Could you check a few things on this model? Use its own coordinates, in mm. Face numbers are marked on the shaded views. A direction names the side the tool comes from. Give positions to 0.01 mm unless a question says otherwise; leave off trailing zeros. Order: outer loops, then holes, each group sorted by start corner. A loop starts at its lowest first (then second) coordinate and runs counter-clockwise, first axis right, second up. Notation, with made-up numbers: (-21.75, 12) - (11.25, 12) arc R19 ccw to (11.25, 23) - close; hole circle Ø9 at (52.5, -8.75). An arc over 180 degrees is marked (long way). Put each result on its own line as item: value.
from build123d import *

# Parameters (mm, degrees)
CYLINDER060_R     = 4
CYLINDER060_DEPTH = 10
BOX018_W          = 6.3
BOX018_H          = 1.8
BOX018_DEPTH      = 14.2
ARRAY003_COUNT    = 16
CYLINDER056_R     = 10.8
CYLINDER056_DEPTH = 14.2
BOX015_W          = 14
BOX015_H          = 54
BOX015_DEPTH      = 15
BOX016_W          = 40
BOX016_H          = 40
BOX016_DEPTH      = 10
PRISM008_DEPTH    = 2.4
PRISM001_DEPTH    = 2.4
CYLINDER012_R     = 1.25
CYLINDER012_DEPTH = 50
CYLINDER011_R     = 1.25
CYLINDER011_DEPTH = 50
CYLINDER007_R     = 6.75
CYLINDER007_DEPTH = 50
CYLINDER008_R     = 6.75
CYLINDER008_DEPTH = 50
BOX013_W          = 18
BOX013_H          = 18
BOX013_DEPTH      = 15
BOX003_W          = 18
BOX003_H          = 18
BOX003_DEPTH      = 15
CYLINDER004_R     = 11.2
CYLINDER004_DEPTH = 23
CYLINDER002_R     = 0.9
CYLINDER002_DEPTH = 19.75
ARRAY002_COUNT    = 10
CYLINDER006_R     = 10.5
CYLINDER006_DEPTH = 32
CYLINDER005_R     = 20
CYLINDER005_DEPTH = 15
FILLET003_R       = 1
CYLINDER051_R     = 1.25
CYLINDER051_DEPTH = 50
BOX011_W          = 16
BOX011_H          = 1
BOX011_DEPTH      = 15
CYLINDER052_R     = 1.25
CYLINDER052_DEPTH = 50
BOX012_W          = 16
BOX012_H          = 1
BOX012_DEPTH      = 15
FILLET010_R       = 0.9
CYLINDER053_R     = 10.5
CYLINDER053_DEPTH = 15
PAD_DEPTH         = 50
BOX014_W          = 10
BOX014_H          = 54
BOX014_DEPTH      = 15
FILLET011_R       = 2


with BuildPart() as cylinder055:
    # Cylinder060 → Cylinder060 (new body)
    with BuildSketch(Plane.XY.offset(21.7)):
        Circle(CYLINDER060_R)
    extrude(amount=CYLINDER060_DEPTH)


with BuildPart() as array003:
    # Box018 → Box018 (new body)
    with BuildSketch(Plane(origin=(6, -0.9, 15), x_dir=(1, 0, 0), z_dir=(0, 0, 1))):
        with Locations((3.15, 0.9)):
            Rectangle(BOX018_W, BOX018_H)
    extrude(amount=BOX018_DEPTH)

    # Array003: Array003 ×16 about axis
    array003_axis = Axis((0, 0, 0), (0, 0, 1))


with BuildPart() as array003_1:
    add(array003.part)
    for i in range(1, ARRAY003_COUNT):
        add(array003.part.rotate(array003_axis, i * 360 / ARRAY003_COUNT))


with BuildPart() as fusion020:
    # Cylinder056 → Cylinder056 (new body)
    with BuildSketch(Plane.XY.offset(15)):
        Circle(CYLINDER056_R)
    extrude(amount=CYLINDER056_DEPTH)

    # Fusion020: union Array003
    add(array003_1.part)


with BuildPart() as cube015:
    # Box015 → Box015 (new body)
    with BuildSketch(Plane(origin=(15, -27, 15), x_dir=(1, 0, 0), z_dir=(0, 0, 1))):
        with Locations((7, 27)):
            Rectangle(BOX015_W, BOX015_H)
    extrude(amount=BOX015_DEPTH)


with BuildPart() as cube016:
    # Box016 → Box016 (new body)
    with BuildSketch(Plane(origin=(-20, -20, 5), x_dir=(1, 0, 0), z_dir=(0, 0, 1))):
        with Locations((20, 20)):
            Rectangle(BOX016_W, BOX016_H)
    extrude(amount=BOX016_DEPTH)


with BuildPart() as prism008:
    # Prism008 → Prism008 (new body)
    with BuildSketch(Plane(origin=(0, 28, 22.5), x_dir=(1, 0, 0), z_dir=(0, -1, 0))):
        Polygon((3.15, 0), (1.575, 2.72798), (-1.575, 2.72798), (-3.15, 0), (-1.575, -2.72798), (1.575, -2.72798), align=None)
    extrude(amount=PRISM008_DEPTH)


with BuildPart() as prism001:
    # Prism001 → Prism001 (new body)
    with BuildSketch(Plane(origin=(0, -25.5, 22.5), x_dir=(1, 0, 0), z_dir=(0, -1, 0))):
        Polygon((3.15, 0), (1.575, 2.72798), (-1.575, 2.72798), (-3.15, 0), (-1.575, -2.72798), (1.575, -2.72798), align=None)
    extrude(amount=PRISM001_DEPTH)


with BuildPart() as cylinder011:
    # Cylinder012 → Cylinder012 (new body)
    with BuildSketch(Plane(origin=(0, 69, 22.5), x_dir=(1, 0, 0), z_dir=(0, -1, 0))):
        Circle(CYLINDER012_R)
    extrude(amount=CYLINDER012_DEPTH)


with BuildPart() as cylinder010:
    # Cylinder011 → Cylinder011 (new body)
    with BuildSketch(Plane(origin=(0, -16, 22.5), x_dir=(1, 0, 0), z_dir=(0, -1, 0))):
        Circle(CYLINDER011_R)
    extrude(amount=CYLINDER011_DEPTH)


with BuildPart() as cylinder007:
    # Cylinder007 → Cylinder007 (new body)
    with BuildSketch(Plane(origin=(-24, 19, 22.5), x_dir=(0, 0, -1), z_dir=(1, 0, 0))):
        Circle(CYLINDER007_R)
    extrude(amount=CYLINDER007_DEPTH)


with BuildPart() as cylinder008:
    # Cylinder008 → Cylinder008 (new body)
    with BuildSketch(Plane(origin=(-24, -19, 22.5), x_dir=(0, 0, -1), z_dir=(1, 0, 0))):
        Circle(CYLINDER008_R)
    extrude(amount=CYLINDER008_DEPTH)


with BuildPart() as cube013:
    # Box013 → Box013 (new body)
    with BuildSketch(Plane(origin=(-9, -29, 15), x_dir=(1, 0, 0), z_dir=(0, 0, 1))):
        with Locations((9, 9)):
            Rectangle(BOX013_W, BOX013_H)
    extrude(amount=BOX013_DEPTH)


with BuildPart() as cube003:
    # Box003 → Box003 (new body)
    with BuildSketch(Plane(origin=(-9, 11, 15), x_dir=(1, 0, 0), z_dir=(0, 0, 1))):
        with Locations((9, 9)):
            Rectangle(BOX003_W, BOX003_H)
    extrude(amount=BOX003_DEPTH)


with BuildPart() as cylinder004:
    # Cylinder004 → Cylinder004 (new body)
    with BuildSketch(Plane.XY):
        Circle(CYLINDER004_R)
    extrude(amount=CYLINDER004_DEPTH)


with BuildPart() as obj1:
    # Cylinder002 → Cylinder002 (new body)
    with BuildSketch(Plane(origin=(0, 0, 15), x_dir=(0, 0, -1), z_dir=(1, 0, 0))):
        Circle(CYLINDER002_R)
    extrude(amount=CYLINDER002_DEPTH)

    # Array002: obj1 ×10 about axis
    array002_axis = Axis((0, 0, 0), (0, 0, 1))


with BuildPart() as obj1_1:
    add(obj1.part)
    for i in range(1, ARRAY002_COUNT):
        add(obj1.part.rotate(array002_axis, i * 360 / ARRAY002_COUNT))

    # Cut002: cut Cylinder004
    add(cylinder004.part, mode=Mode.SUBTRACT)


with BuildPart() as cylinder006:
    # Cylinder006 → Cylinder006 (new body)
    with BuildSketch(Plane.XY):
        Circle(CYLINDER006_R)
    extrude(amount=CYLINDER006_DEPTH)


with BuildPart() as obj2:
    # Cylinder005 → Cylinder005 (new body)
    with BuildSketch(Plane.XY.offset(15)):
        Circle(CYLINDER005_R)
    extrude(amount=CYLINDER005_DEPTH)

    # Cut004: cut Cylinder006
    add(cylinder006.part, mode=Mode.SUBTRACT)

    # Fusion001: union obj1
    add(obj1_1.part)

    # Fusion002: union Cube013, Cube003
    add(cube013.part)
    add(cube003.part)

    # Cut005: cut Cylinder008
    add(cylinder008.part, mode=Mode.SUBTRACT)

    # Cut006: cut Cylinder007
    add(cylinder007.part, mode=Mode.SUBTRACT)

    # Fillet003
    fillet003_edges = [obj2.edges().sort_by_distance(p)[0] for p in [
        (-9, -17.860571, 29.576567),
        (-9, -17.860571, 15.423433),
        (-9, -29, 22.5),
        (-9, 17.860571, 15.423433),
        (-9, 17.860571, 29.576567),
        (9, -29, 22.5),
        (9, -17.860571, 29.576567),
        (9, -17.860571, 15.423433),
        (9, 17.860571, 29.576567),
        (9, 17.860571, 15.423433),
        (9, 29, 22.5),
        (-9, 29, 22.5),
    ]]
    fillet(fillet003_edges, radius=FILLET003_R)

    # Cut008: cut Cylinder010
    add(cylinder010.part, mode=Mode.SUBTRACT)

    # Cut009: cut Cylinder011
    add(cylinder011.part, mode=Mode.SUBTRACT)

    # Cut035: cut Prism001
    add(prism001.part, mode=Mode.SUBTRACT)

    # Cut036: cut Prism008
    add(prism008.part, mode=Mode.SUBTRACT)


with BuildPart() as cylinder049:
    # Cylinder051 → Cylinder051 (new body)
    with BuildSketch(Plane(origin=(0, 69, 22.5), x_dir=(1, 0, 0), z_dir=(0, -1, 0))):
        Circle(CYLINDER051_R)
    extrude(amount=CYLINDER051_DEPTH)


with BuildPart() as cut037:
    # Box011 → Box011 (new body)
    with BuildSketch(Plane(origin=(-8, 29, 15), x_dir=(1, 0, 0), z_dir=(0, 0, 1))):
        with Locations((8, 0.5)):
            Rectangle(BOX011_W, BOX011_H)
    extrude(amount=BOX011_DEPTH)

    # Cut037: cut Cylinder049
    add(cylinder049.part, mode=Mode.SUBTRACT)


with BuildPart() as cylinder021:
    # Cylinder052 → Cylinder052 (new body)
    with BuildSketch(Plane(origin=(0, 69, 22.5), x_dir=(1, 0, 0), z_dir=(0, -1, 0))):
        Circle(CYLINDER052_R)
    extrude(amount=CYLINDER052_DEPTH)


with BuildPart() as obj3:
    # Box012 → Box012 (new body)
    with BuildSketch(Plane(origin=(-8, 29, 15), x_dir=(1, 0, 0), z_dir=(0, 0, 1))):
        with Locations((8, 0.5)):
            Rectangle(BOX012_W, BOX012_H)
    extrude(amount=BOX012_DEPTH)

    # Cut038: cut Cylinder021
    add(cylinder021.part, mode=Mode.SUBTRACT)


with BuildPart() as obj3_1:
    # Cut038 placement: moved
    add(obj3.part.moved(Location((0, -59, 0))))

    # Fusion017: union obj2, Cut037
    add(obj2.part)
    add(cut037.part)

    # Fillet010
    fillet010_edges = [obj3_1.edges().sort_by_distance(p)[0] for p in [
        (-8, -30, 22.5),
        (8, -30, 22.5),
        (-8, 30, 22.5),
        (8, 30, 22.5),
    ]]
    fillet(fillet010_edges, radius=FILLET010_R)


with BuildPart() as cylinder050:
    # Cylinder053 → Cylinder053 (new body)
    with BuildSketch(Plane.XY.offset(15)):
        Circle(CYLINDER053_R)
    extrude(amount=CYLINDER053_DEPTH)


with BuildPart() as body:
    # CopySketch → Pad (new body)
    with BuildSketch(Plane(origin=(0, 0, 15), x_dir=(1, 0, 0), z_dir=(0, 0, -1))):
        with BuildLine():
            Line((9, 28), (9, 18.466185))
            ThreePointArc((9, 18.466185), (9.140875, 17.954419), (9.52381, 17.586843))
            ThreePointArc((9.52381, -17.586843), (20, 0), (9.52381, 17.586843))
            ThreePointArc((9.52381, -17.586843), (9.140875, -17.954419), (9, -18.466185))
            Line((9, -18.466185), (9, -28))
            Line((27.474319, -28), (9, -28))
            Line((27.474319, 28), (27.474319, -28))
            Line((9, 28), (27.474319, 28))
        make_face()
    extrude(amount=PAD_DEPTH)


with BuildPart() as body_1:
    # Body placement: moved
    add(body.part.moved(Location((0, 0, 25))))


with BuildPart() as obj4:
    # Box014 → Box014 (new body)
    with BuildSketch(Plane(origin=(7, -27, 15), x_dir=(1, 0, 0), z_dir=(0, 0, 1))):
        with Locations((5, 27)):
            Rectangle(BOX014_W, BOX014_H)
    extrude(amount=BOX014_DEPTH)

    # Cut039: cut Body
    add(body_1.part, mode=Mode.SUBTRACT)

    # Fusion018: union Cylinder050
    add(cylinder050.part)

    # Fusion019: union obj3
    add(obj3_1.part)

    # Cut040: cut Cube016
    add(cube016.part, mode=Mode.SUBTRACT)

    # Cut041: cut Cube015
    add(cube015.part, mode=Mode.SUBTRACT)

    # Fillet011
    fillet011_edges = [obj4.edges().sort_by_distance(p)[0] for p in [
        (15, 13.228757, 28.000375),
        (15, 13.228757, 22.5),
        (15, 13.228757, 16.999625),
        (15, -13.228757, 16.999625),
        (15, -13.228757, 22.5),
        (15, -13.228757, 28.000375),
    ]]
    fillet(fillet011_edges, radius=FILLET011_R)

    # Cut042: cut Fusion020
    add(fusion020.part, mode=Mode.SUBTRACT)

    # Cut045: cut Cylinder055
    add(cylinder055.part, mode=Mode.SUBTRACT)


solid = obj4.part
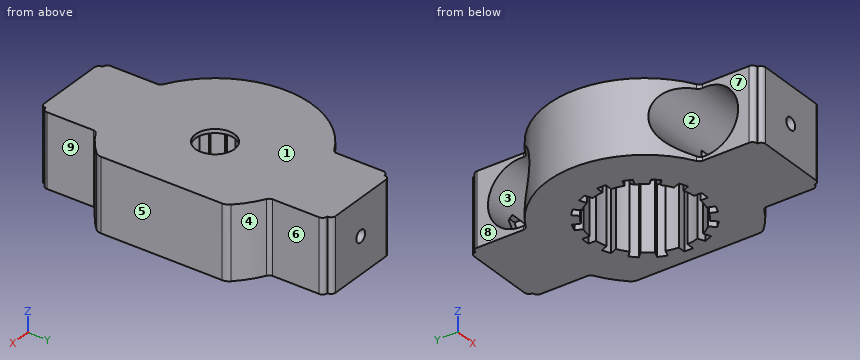
1) Which directions (+Z, -Z, +X, -X, +Y, -Y) give clear straight access to the entire face, cutting with the end or side of a thin tool? Please do the marked faces 5, 6, 7, 8 and 9.
Filled in:
face 5: +Z, -Z, +X, +Y, -Y
face 6: +Z, -Z, +X, +Y
face 7: +Z, -Z, -X, -Y
face 8: +Z, -Z, -X, +Y
face 9: +Z, -Z, +X, -Y
2) Suppose I cut it at C-C, the plane x = -16.5. List the corners of the cut face in (y, z) for me.
Filled in:
outline: (-11.3, 15) - (11.3, 15) - (11.3, 30) - (-11.3, 30) - close
3) Suppose I cut it at A-A, the plane y = 26.5. List the corners of the cut face in (x, z) for me (3 decimals).
Filled in:
outline: (-9, 15) - (9, 15) - (9, 30) - (-9, 30) - close; hole (-3.15, 22.5) - (-1.575, 19.772) - (1.575, 19.772) - (3.15, 22.5) - (1.575, 25.228) - (-1.575, 25.228) - close
4) We'd pull the mould along Y, two halves only. Please class the marked faces 1, 2, 3 and 4: pulls with the +Y half, pulls with the -Y half, needs draft (parallel to the pull), parting line crosses it, or undercut.
Filled in:
face 1: needs draft
face 2: undercut
face 3: undercut
face 4: pulls with the +Y half
5) Suppose I cut it at B-B, the plane y = 0. List the corners of the cut face in (x, z) for me.
Filled in:
outline: (-20, 15) - (-12.3, 15) - (-12.3, 29.2) - (-4, 29.2) - (-4, 30) - (-20, 30) - close; (4, 29.2) - (12.3, 29.2) - (12.3, 15) - (15, 15) - (15, 30) - (4, 30) - close
6) If I drill on line 1 (Y direction, x = 1.5, z = 19.5); line 2 (Y direction, x = 0, z = 29.6); line 3 (Y direction, x = -4, z = 22), over which ranges is the centre line in solid material (lowest first)? Write a range as [from, to].
Filled in:
line 1: y = [-30, -25.05], [-12.95, -10.7], [10.7, 12.95], [25.05, 30]
line 2: y = [-30, -4], [4, 30]
line 3: y = [-30, -25.73], [-12.27, -11.66], [11.66, 12.27], [25.73, 30]
7) I'm going to push flat-ended pins straight in: pin 1 (2 mm diameter, centred on y = 23.5, z = 26, fed in from +X); pin 2 (7.5 mm diameter, centred on y = 25, z = 22.5, fed in from -X); pin 3 (1.7 mm diameter, centred on x = -11, z = 21, fed in from +Y); pin 4 (6.5 mm diameter, centred on x = 0, y = 0, fed in from -Z). Where does each tip first touch, or does it pass through?
Filled in:
pin 1: stops at x = 9
pin 2: stops at x = -9
pin 3: stops at y = 12.67
pin 4: passes through
